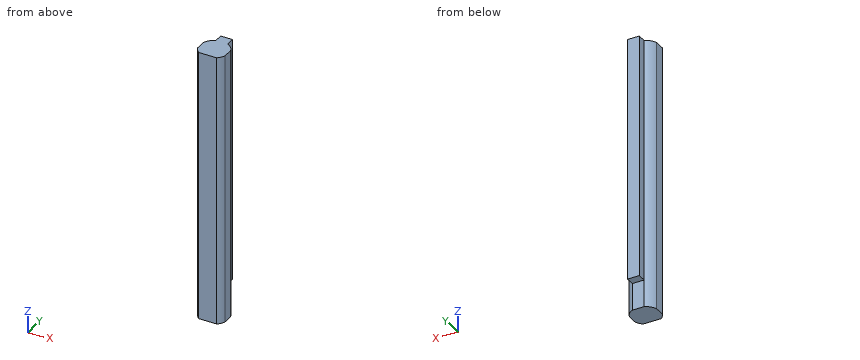
from build123d import *

# Parameters (mm, degrees)
BOSS_EXTRUDE1_DEPTH = 150
BOSS_EXTRUDE2_START = 150
SKETCH1_3_W         = 6.5
SKETCH1_3_H         = 4.689904241
BOSS_EXTRUDE2_DEPTH = 135


with BuildPart() as part:
    # Sketch1 → Boss-Extrude1 (new body)
    with BuildSketch(Plane.XY):
        with BuildLine():
            Line((3.25, 7.310095759), (-3.25, 7.310095759))
            ThreePointArc((-3.25, 7.310095759), (-5.832004573, 5.476104698), (-7.5, 2.783882181))
            Line((-7.5, 2.783882181), (-7.5, -2.783882181))
            ThreePointArc((-7.5, -2.783882181), (-6.466277075, -4.710335529), (-4.949623723, -6.285))
            Line((-4.949623723, -6.285), (4.949623723, -6.285))
            ThreePointArc((4.949623723, -6.285), (6.466277075, -4.710335529), (7.5, -2.783882181))
            Line((7.5, -2.783882181), (7.5, 2.783882181))
            ThreePointArc((7.5, 2.783882181), (5.832004573, 5.476104698), (3.25, 7.310095759))
        make_face()
    extrude(amount=BOSS_EXTRUDE1_DEPTH)

    # Sketch1<3> → Boss-Extrude2 (add)
    with BuildSketch(Plane.XY.offset(BOSS_EXTRUDE2_START)):
        with Locations((0, 9.655047879)):
            Rectangle(SKETCH1_3_W, SKETCH1_3_H)
    extrude(amount=-BOSS_EXTRUDE2_DEPTH)


solid = part.part
Part model, mm, in its own coordinate system. Give positions to 0.01 mm unless a question says otherwise; leave off trailing zeros. Order: outer loops, then holes, each group sorted by start corner. A loop starts at its lowest first (then second) coordinate and runs counter-clockwise, first axis right, second up. Notation, with made-up numbers: (1, 24) - (30, 24) arc R21 ccw to (30, 30) - close; hole circle Ø5 at (62, -23.5). An arc over 180 degrees is marked (long way). Use a Markdown table: item, result.
1) Probe L1, parallel to X at y = 11.25, z = 73; L2, parallel to X at y = 4.25, z = 22; L3, parallel to Y at x = -6, z = 81. List the from-to ranges inside material, lowest first. Write a range as from..to.
Checked values:
| item | result |
|---|---|
| L1 | -3.25..3.25 |
| L2 | -6.78..6.78 |
| L3 | -5.29..5.29 |
2) Saw through at B-B on x = 0. List the corners of the cut face in (y, z) (3 decimals), plus the area to 3 significant figures.
Checked values:
| item | result |
|---|---|
| outline | (-6.285, 0) - (7.31, 0) - (7.31, 15) - (12, 15) - (12, 150) - (-6.285, 150) - close |
| area | 2,670 mm² |
3) Flat gauge pins, fed straight in: P1, Ø7, axis at x = 0, z = 7, coming from the +Y side; P2, Ø4, axis at x = -1.5, y = 9.5, coming from the -Z side; P3, Ø5, axis at y = 10.5, z = 84, coming from the +X side. Where does each tip first touch, or does it go through?
Checked values:
| item | result |
|---|---|
| P1 | y = 7.31 |
| P2 | z = 15 |
| P3 | x = 3.25 |
4) Saw through at C-C on y = -4.75. List the corners of the cut face in (x, z), plus the area to 3 significant figures.
Checked values:
| item | result |
|---|---|
| outline | (-6.44, 0) - (6.44, 0) - (6.44, 150) - (-6.44, 150) - close |
| area | 1,930 mm² |
5) Saw through at A-A on z = 52.5. List the corners of the cut face in (x, y) (3 decimals).
Checked values:
| item | result |
|---|---|
| outline | (-7.5, -2.784) arc R8 ccw to (-4.95, -6.285) - (4.95, -6.285) arc R8 ccw to (7.5, -2.784) - (7.5, 2.784) arc R8 ccw to (3.25, 7.31) - (3.25, 12) - (-3.25, 12) - (-3.25, 7.31) arc R8 ccw to (-7.5, 2.784) - close |
